For this review, use the dimensioned drawing (mm, ordinates from the lowest corner) and the shaded views. Coordinates: 2 decimals unless noted, no trailing zeros. Loops run counter-clockwise (first coordinate to the right, second up) from the corner with the lowest first, then second, coordinate; pieces in that order, holes last. Notation, with made-up numbers: M 0.5,51.5 L 21.5,51.5 A23 ccw 21.5,64.5 Z; hole C 30,85.5 d10. An arc over 180 degrees is marked long. Use CSV: the item, a comma, the result in double quotes. Start each with the question number.
1. Add section D-D, the plane z = 0.95. Write out the cut boundary in (x, y) (3 decimals).
2. Add section A-A, the plane x = 22. Write out the cut boundary in (y, z).
3. Add section B-B, the plane y = 22. Write out the cut boundary in (x, z).
4. For L1, parallel to Y at x = 22, z = 0.75; L2, parallel to Y at x = 20.5, z = 1.2; L3, parallel to Y at x = 20, z = 1.3, list the stretches that pass through material, from the lowest coordinate up.
5. Add section C-C, the plane x = 28.5. Write out the cut boundary in (y, z).
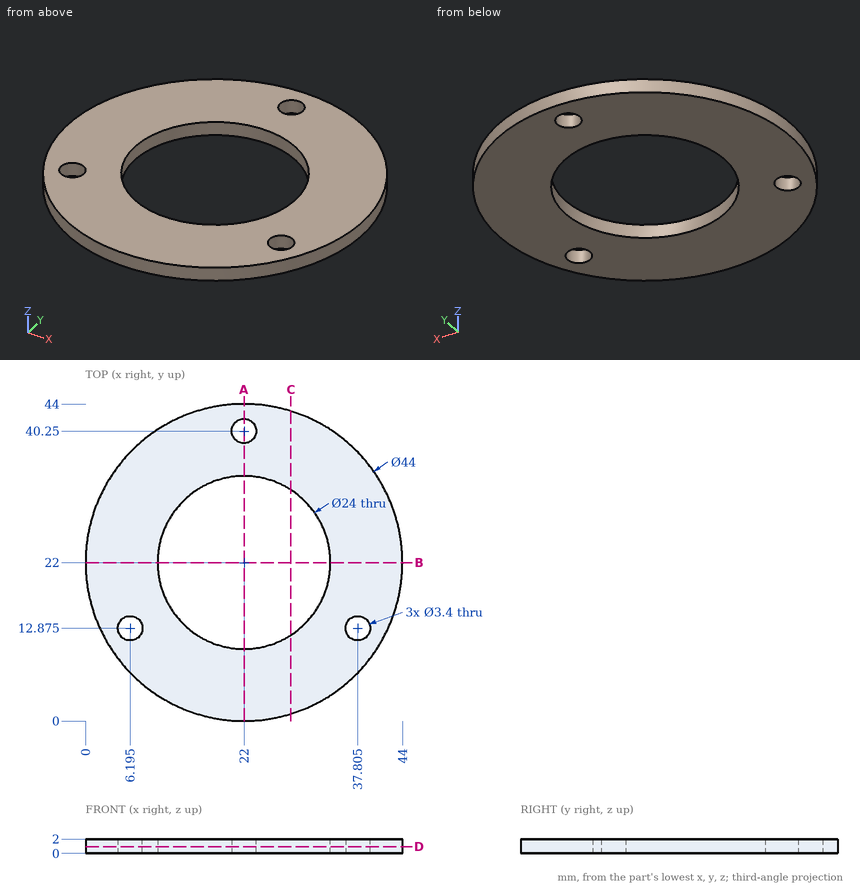
Computed:
1,outline,"C 22,22 d44; hole C 6.195,12.875 d3.4; hole C 22,22 d24; hole C 22,40.25 d3.4; hole C 37.805,12.875 d3.4"
2,outline,"M 0,0 L 10,0 L 10,2 L 0,2 Z; M 34,0 L 38.55,0 L 38.55,2 L 34,2 Z; M 41.95,0 L 44,0 L 44,2 L 41.95,2 Z"
3,outline,"M 0,0 L 10,0 L 10,2 L 0,2 Z; M 34,0 L 44,0 L 44,2 L 34,2 Z"
4,L1,"y = 0 to 10, 34 to 38.55, 41.95 to 44"
4,L2,"y = 0.05 to 10.09, 33.91 to 39.45, 41.05 to 43.95"
4,L3,"y = 0.09 to 10.17, 33.83 to 43.91"
5,outline,"M 0.98,0 L 11.91,0 L 11.91,2 L 0.98,2 Z; M 32.09,0 L 43.02,0 L 43.02,2 L 32.09,2 Z"
